from build123d import *

# Parameters (mm, degrees)
BOSS_EXTRUDE1_DEPTH             = 60
BOSS_EXTRUDE2_DEPTH             = 35
CUT_EXTRUDE1_DEPTH              = 103.668316888
CUT_EXTRUDE2_DEPTH              = 113.568195388
CUT_EXTRUDE3_DEPTH              = 112.060037393
BOSS_EXTRUDE3_DEPTH             = 5
BOSS_EXTRUDE3_DIRECTION_2_REACH = 115.625
BOSS_EXTRUDE4_DEPTH             = 3.2
BOSS_EXTRUDE5_DEPTH             = 28.5
BOSS_EXTRUDE6_DEPTH             = 3.2
SKETCH8_W                       = 25.2
SKETCH8_H                       = 32.67766953
CUT_EXTRUDE4_DEPTH              = 111.954500313
CHAMFER1_SIZE                   = 0.8
FILLET1_R                       = 5
FILLET2_R                       = 3
FILLET3_R                       = 3
CHAMFER2_SIZE                   = 1.6
CHAMFER3_SIZE                   = 0.8


with BuildPart() as part:
    # Sketch1 → Boss-Extrude1 (new body)
    with BuildSketch(Plane(origin=(0, 0, 0), x_dir=(0, 0, -1), z_dir=(1, 0, 0))):
        Polygon((-9, 9.5), (13, 9.5), (13, -19), (-9, -19), (-9, -22.2), (13, -22.2), (13, -37.2), (-3.07766953, -53.27766953), (-1.47766953, -54.87766953), (16.2, -37.2), (16.2, 12.7), (-10.847520861, 12.7), (-17.256108849, 1.6), (-14.484827557, 0), align=None)
    extrude(amount=BOSS_EXTRUDE1_DEPTH)

    # Sketch2 → Boss-Extrude2 (add)
    with BuildSketch(Plane(origin=(60, 0, 0), x_dir=(0, 0, -1), z_dir=(1, 0, 0))):
        Polygon((-3.07766953, -53.27766953), (-1.47766953, -54.87766953), (16.2, -37.2), (16.2, 12.7), (13, 12.7), (13, -37.2), align=None)
    extrude(amount=BOSS_EXTRUDE2_DEPTH)

    # Sketch3 → Cut-Extrude1 (cut, through all)
    with BuildSketch(Plane.XZ.offset(22.2)):
        Polygon((60, -13), (42.531627411, 17.256108849), (60, 17.256108849), align=None)
    extrude(amount=-CUT_EXTRUDE1_DEPTH, mode=Mode.SUBTRACT)

    # Sketch4 → Cut-Extrude2 (cut, through all)
    with BuildSketch(Plane.XY.offset(9)):
        Polygon((47.298294078, 9.5), (37.798294078, 0), (47.298294078, 0), align=None)
    extrude(amount=CUT_EXTRUDE2_DEPTH, mode=Mode.SUBTRACT)

    # Sketch5 → Cut-Extrude3 (cut, through all)
    with BuildSketch(Plane.ZY):
        Polygon((16.563288526, 2.8), (16.563288526, 1.2), (17.256108849, 1.6), align=None)
        Polygon((2.27766953, -52.47766953), (2.27766953, -54.07766953), (3.07766953, -53.27766953), align=None)
    extrude(amount=-CUT_EXTRUDE3_DEPTH, mode=Mode.SUBTRACT)

    # Sketch6 → Boss-Extrude3 (add)
    with BuildSketch(Plane.XY.offset(-13)):
        Polygon((78.8, 13), (91.8, 13), (91.8, -13), (78.8, -13), (78.8, -16.2), (95, -16.2), (95, 16.2), (78.8, 16.2), align=None)
    extrude(amount=BOSS_EXTRUDE3_DEPTH)

    # Boss-Extrude3 direction 2: up to this face of the body (flat: up to its plane)
    boss_extrude3_direction_2_end = Plane(part.part.faces().sort_by_distance((47.5, -12.25, -16.2))[0])
    # Sketch6 → Boss-Extrude3 direction 2 (add, up to the picked face)
    with BuildSketch(Plane.XY.offset(-13), mode=Mode.PRIVATE) as boss_extrude3_direction_2_sk1:
        Polygon((78.8, 13), (91.8, 13), (91.8, -13), (78.8, -13), (78.8, -16.2), (95, -16.2), (95, 16.2), (78.8, 16.2), align=None)
    boss_extrude3_direction_2_tool1 = split(extrude(boss_extrude3_direction_2_sk1.sketch, amount=-BOSS_EXTRUDE3_DIRECTION_2_REACH, mode=Mode.PRIVATE), bisect_by=boss_extrude3_direction_2_end, keep=Keep.BOTH, mode=Mode.PRIVATE)
    add(boss_extrude3_direction_2_tool1.solids().sort_by(Axis((85.3, 13.362243, -13), (0, 0, -1)))[0])

    # Sketch7 → Boss-Extrude4 (add)
    with BuildSketch(Plane(origin=(0, 0, -16.2), x_dir=(-1, 0, 0), z_dir=(0, 0, -1))):
        Polygon((-95, 16.2), (-78.8, 16.2), (-75.3, 12.7), (-95, 12.7), align=None)
    extrude(amount=-BOSS_EXTRUDE4_DEPTH)

    # Sketch9 → Boss-Extrude5 (add)
    with BuildSketch(Plane(origin=(0, -19, 0), x_dir=(1, 0, 0), z_dir=(0, 1, 0))):
        Polygon((33.798294078, 9), (37.798294078, 13), (0, 13), (0, 9), align=None)
    extrude(amount=BOSS_EXTRUDE5_DEPTH)

    # Sketch10 → Boss-Extrude6 (add)
    with BuildSketch(Plane.ZY):
        Polygon((6.5, -19), (-3, -9.5), (-9, -9.5), (-9, -19), align=None)
    extrude(amount=-BOSS_EXTRUDE6_DEPTH)

    # Sketch8 → Cut-Extrude4 (cut, through all)
    with BuildSketch(Plane.ZY):
        with Locations((-3.6, -38.538834765)):
            Rectangle(SKETCH8_W, SKETCH8_H)
    extrude(amount=-CUT_EXTRUDE4_DEPTH, mode=Mode.SUBTRACT)

    # Chamfer1
    chamfer1_edges = [part.edges().sort_by_distance(p)[0] for p in [
        (78.8, 14.6, -8),
        (85.3, 13, -8),
        (91.8, 0, -8),
        (85.3, -13, -8),
        (78.8, -14.6, -8),
        (86.9, -16.2, -8),
        (95, 0, -8),
        (86.9, 16.2, -8),
    ]]
    chamfer(chamfer1_edges, length=CHAMFER1_SIZE)

    # Fillet1
    # the kernel refuses this fillet: 5 mm, written as the material it adds along each edge
    with BuildSketch(Plane(origin=(78.8, -16.2, -13), x_dir=(0, 0, 1), z_dir=(1, 0, 0))) as fillet1_piece_1:
        with BuildLine():
            CenterArc((5, 4.935585072), FILLET1_R, 180, 80.793103779)
            Line((0, 4.935585072), (0, 0))
            Line((0, 0), (4.2, 0))
        make_face()
    extrude(amount=16.2)

    # Fillet2
    fillet2_edges = [part.edges().sort_by_distance(p)[0] for p in [
        (35.798294078, -19, -11),
        (16.899147039, 9.5, -9),
        (35.798294078, 9.5, -11),
        (18.499147039, -19, -9),
        (1.6, -9.5, -9),
        (48.899147039, 9.5, -13),
        (48.899147039, -19, -13),
    ]]
    fillet(fillet2_edges, radius=FILLET2_R)

    # Fillet3
    fillet3_edges = [part.edges().sort_by_distance(p)[0] for p in [
        (3.2, -19, 0.25),
        (3.2, -11.25, -9),
        (3.2, -18.121320344, -8.121320344),
    ]]
    fillet(fillet3_edges, radius=FILLET3_R)

    # Chamfer2
    chamfer2_edges = [part.edges().sort_by_distance(p)[0] for p in [
        (86.9, 16.2, -16.2),
        (37.65, 12.7, -16.2),
        (77.05, 14.45, -16.2),
        (95, -3, -16.2),
        (0, -4.75, -16.2),
        (47.5, -22.2, -16.2),
    ]]
    chamfer(chamfer2_edges, length=CHAMFER2_SIZE)

    # Chamfer3
    chamfer3_edges = [part.edges().sort_by_distance(p)[0] for p in [
        (23.649147039, -22.2, 9),
        (23.649147039, -19, 9),
    ]]
    chamfer(chamfer3_edges, length=CHAMFER3_SIZE)


solid = part.part
The listing builds one solid part. Answer for the finished solid, in the listing's coordinates (mm). A direction names the side the tool comes from. Give positions to 0.01 mm unless a question says otherwise; leave off trailing zeros. Order: outer loops, then holes, each group sorted by start corner. A loop starts at its lowest first (then second) coordinate and runs counter-clockwise, first axis right, second up. Notation, with made-up numbers: (1, 50) - (12, 50) arc R5 cw to (12, 55) - close; hole circle Ø9 at (-21.5, 29.5). An arc over 180 degrees is marked (long way). Answer as CSV lines item,"result".
Q1. Each of these flat-tipped pins is pushed along its axis until it touches: pin 1 Ø1.6 at (y, z) = (14.5, -11.5) entering from -X; pin 2 Ø0.5 at (x, y) = (31, -20.5) entering from +Z; pin 3 Ø14.5 at (x, z) = (39.5, -1) entering from +Y; pin 4 Ø3.5 at (x, z) = (83, -11.5) entering from -Y. Where does it stop, or does it pass through?
Answer key:
pin 1,"stops at x = 78.8"
pin 2,"stops at z = 9"
pin 3,"stops at y = 12.7"
pin 4,"stops at y = -22.2"
Q2. Straight lines are drawn through the part: L1, parallel to Y at x = 8, z = 0; L2, parallel to Z at x = 19, y = -2.5; L3, parallel to Z at x = 64, y = 5.5. For each, find the intervals that lie inside material, in ascending order.
Answer key:
L1,"y = -22.2 to -19, 9.5 to 12.7"
L2,"z = -16.2 to -9"
L3,"z = -16.2 to -13"
Q3. Which of the six approach directions +Z, -Z, +X, -X, +Y, -Y give full straight-line access (tool end or side, diameter ignored) to faces 5 (the face through (91.8, 0, -11)), 6 (the face through (78.8, -15, -11)), 7 (the face through (36.03, 8.64, -9.96))?
Answer key:
face 5,"+Z"
face 6,"+Z, +Y, -Y"
face 7,"none"
Q4. A cutting plane is placed at D-D, the plane y = -10.5. Determine the outline of the cut face in (x, z).
Answer key:
outline,"(0, -14.6) - (1.6, -16.2) - (93.4, -16.2) - (95, -14.6) - (95, -8.8) - (94.2, -8) - (92.6, -8) - (91.8, -8.8) - (91.8, -13) - (37.8, -13) - (33.8, -9) - (6.2, -9) arc R3 cw to (3.2, -6) - (3.2, -2) - (0, -2) - close"
Q5. A cutting plane is placed at A-A, the plane x = 84. Determine the outline of the cut face in (y, z), and give its area (3 significant figures).
Answer key:
outline,"(-22.2, -14.6) - (-20.6, -16.2) - (14.6, -16.2) - (16.2, -14.6) - (16.2, -8.8) - (15.4, -8) - (13.8, -8) - (13, -8.8) - (13, -13) - (-13, -13) - (-13, -8.8) - (-13.8, -8) - (-15.4, -8) - (-16.2, -8.8) arc R5 cw to (-21.14, -13) - (-22.2, -13) - close"
area,"156 mm^2"
Q6. A cutting plane is placed at B-B, the plane z = 0. Determine the outline of the cut face in (x, y), and give its area (3 significant figures).
Answer key:
outline,"(0, -22.2) - (52.49, -22.2) - (52.49, -19) - (6.2, -19) arc R3 cw to (3.2, -16) - (3.2, -12.5) - (0, -12.5) - close; (0, 9.5) - (52.49, 9.5) - (52.49, 12.7) - (0, 12.7) - close"
area,"359 mm^2"
Q7. Determine the mould class of faces 1 (the face through (29, -19, 1)), 2 (the face through (4.06, -12.37, -8.1)), 3 (the face through (17.77, 8.64, -8.1)), 4 (the face through (48, -3, -16.2)) for opening direction Z: pulls with the +Z half, pulls with the -Z half, needs draft (parallel to the pull), parting line crosses it, or undercut.
Answer key:
face 1,"needs draft"
face 2,"pulls with the +Z half"
face 3,"undercut"
face 4,"pulls with the -Z half"
Q8. A cutting plane is placed at C-C, the plane y = 4. Determine the outline of the cut face in (x, z).
Answer key:
outline,"(0, -14.6) - (1.6, -16.2) - (93.4, -16.2) - (95, -14.6) - (95, -8.8) - (94.2, -8) - (92.6, -8) - (91.8, -8.8) - (91.8, -13) - (37.8, -13) - (33.8, -9) - (0, -9) - close; (0, 12.18) - (41.8, 12.18) - (41.8, 15.87) - (0, 15.87) - close"
